from build123d import *

# Parameters (mm, degrees)
SKETCH2_R            = 111.5
SKETCH2_R_2          = 14
BOSS_EXTRUDE1_DEPTH  = 5
M4_CLEARANCE_HOLE2_D = 4.5
CUT_EXTRUDE1_DEPTH   = 6


with BuildPart() as part:
    # Sketch2 → Boss-Extrude1 (new body)
    with BuildSketch(Plane(origin=(0, 0, 0), x_dir=(1, 0, 0), z_dir=(0, 1, 0))):
        Circle(SKETCH2_R)
        Circle(SKETCH2_R_2, mode=Mode.SUBTRACT)
    extrude(amount=BOSS_EXTRUDE1_DEPTH)

    # M4 Clearance Hole2 (through all)
    with Locations(Plane(origin=(0, 5, 0), x_dir=(1, 0, 0), z_dir=(0, 1, 0))):
        with Locations((-90.932667397, -52.5), (90.932667397, -52.5), (0, 105)):
            Hole(M4_CLEARANCE_HOLE2_D / 2)

    # Sketch8 → Cut-Extrude1 (cut, through all)
    with BuildSketch(Plane(origin=(0, 5, 0), x_dir=(1, 0, 0), z_dir=(0, 1, 0))):
        with BuildLine():
            Line((-30, 40), (-30, 107.388314076))
            ThreePointArc((-30, 107.388314076), (-96.561832522, 55.75), (-108.001008059, -27.713394924))
            Line((-108.001008059, -27.713394924), (-49.641016151, 5.980762114))
            ThreePointArc((-49.641016151, 5.980762114), (-43.301270189, 25), (-30, 40))
        make_face()
        with BuildLine():
            Line((30, 40), (30, 107.388314076))
            ThreePointArc((30, 107.388314076), (96.561832522, 55.75), (108.001008059, -27.713394924))
            Line((108.001008059, -27.713394924), (49.641016151, 5.980762114))
            ThreePointArc((49.641016151, 5.980762114), (43.301270189, 25), (30, 40))
        make_face()
        with BuildLine():
            Line((19.641016151, -45.980762114), (78.001008059, -79.674919151))
            ThreePointArc((78.001008059, -79.674919151), (0, -111.5), (-78.001008059, -79.674919151))
            Line((-78.001008059, -79.674919151), (-19.641016151, -45.980762114))
            ThreePointArc((-19.641016151, -45.980762114), (0, -50), (19.641016151, -45.980762114))
        make_face()
    extrude(amount=-CUT_EXTRUDE1_DEPTH, mode=Mode.SUBTRACT)


solid = part.part
Source: CAD feature listing. Evaluate the final solid. Frame: model axes, mm. A direction names the side the tool comes from. Round coordinates to 2 decimals unless told otherwise and drop trailing zeros. Order: outer loops, then holes, each group sorted by start corner. A loop starts at its lowest first (then second) coordinate and runs counter-clockwise, first axis right, second up. Notation, with made-up numbers: (-40, -11.75) - (2, -11.75) arc R11 cw to (2, 2.25) - close; hole circle Ø11 at (72.5, -15). An arc over 180 degrees is marked (long way). Use a Markdown table: item, result. Add a question column.
1. Set-up query: faces 1 (the flat face through (30, 3, -73)), 2 (the flat face through (-49.23, 2.535, 63.064)), 3 (the flat face through (-30, 3, -73)), 4 (the cylindrical face through (12.932, 2.465, 5.362)), 5 (the flat face through (-2, 0, -17)). Return all of +Z, -Z, +X, -X, +Y, -Y with unobstructed straight access to the full face (end or side cutting, diameter ignored); none if empty.
2. Section query C-C (z = -57.5). Return the cut outline in (x, y), then the cut area to 3 significant figures.
3. Line query: probe 1 along Z at (x, y) = (0, 1.95); probe 2 along X at (y, z) = (1.1, 52.5); probe 3 along X at (y, z) = (3.15, 64). Output: solid intervals per line, ascending.
4. Mould query, pull axis Z, two halves, no side actions, for faces 6 (the cylindrical face through (-92.14, 2.46, 50.6)), 7 (the flat face through (-79.23, 2.535, 11.102)), 8 (the flat face through (48.41, 2.54, 62.59)). Classes: +Z half, -Z half, draft (parallel to the pull), parting line (faces both ways), or undercut.
5. First-contact query: pin 1 (1.5 mm diameter, centred on x = -39.5, y = 3, fed in from -Z); pin 2 (1.5 mm diameter, centred on y = 2, z = -77, fed in from +X); pin 3 (3 mm diameter, centred on x = 8, y = 1, fed in from -Z); pin 4 (7 mm diameter, centred on x = 90.93, z = 52.5, fed in from +Y). Flat tips, straight axial feed; report the tip coordinate or a pass-through.
6. Section query D-D (x = 45). Return the cut outline in (y, z), then the cut area to 3 significant figures.
7. Section query B-B (y = 3.8). Return the cut outline in (x, z).
8. Section query A-A (z = 0). Return the cut outline in (x, y), then the cut area to 3 significant figures.
Derived:
| question | item | result |
|---|---|---|
| 1 | face 1 | -Z, +X, +Y, -Y |
| 1 | face 2 | +Z, +Y, -Y |
| 1 | face 3 | -Z, -X, +Y, -Y |
| 1 | face 4 | +Y, -Y |
| 1 | face 5 | +Z, -Z, +X, -X, -Y |
| 2 | outline | (-30, 0) - (30, 0) - (30, 5) - (-30, 5) - close |
| 2 | area | 300 mm2 |
| 3 | probe 1 | -111.5 to -107.25, -102.75 to -14, 14 to 50 |
| 3 | probe 2 | -98.37 to -93.18, -88.68 to -30.93, 30.93 to 88.68, 93.18 to 98.37 |
| 3 | probe 3 | -91.3 to -50.85, 50.85 to 91.3 |
| 4 | face 6 | undercut |
| 4 | face 7 | -Z half |
| 4 | face 8 | +Z half |
| 5 | pin 1 | z = -31.6 |
| 5 | pin 2 | x = 30 |
| 5 | pin 3 | z = -111.31 |
| 5 | pin 4 | y = 5 |
| 6 | outline | (0, -21.79) - (5, -21.79) - (5, 60.62) - (0, 60.62) - close |
| 6 | area | 412 mm2 |
| 7 | outline | (-108, 27.71) - (-49.64, -5.98) arc R50 ccw to (-30, -40) - (-30, -107.39) arc R111.5 ccw to (30, -107.39) - (30, -40) arc R50 ccw to (49.64, -5.98) - (108, 27.71) arc R111.5 ccw to (78, 79.67) - (19.64, 45.98) arc R50 ccw to (-19.64, 45.98) - (-78, 79.67) arc R111.5 ccw to start; hole circle Ø4.5 at (-90.93, 52.5); hole circle Ø28 at (0, 0); hole circle Ø4.5 at (0, -105); hole circle Ø4.5 at (90.93, 52.5) |
| 8 | outline | (-60, 0) - (-14, 0) - (-14, 5) - (-60, 5) - close; (14, 0) - (60, 0) - (60, 5) - (14, 5) - close |
| 8 | area | 460 mm2 |
